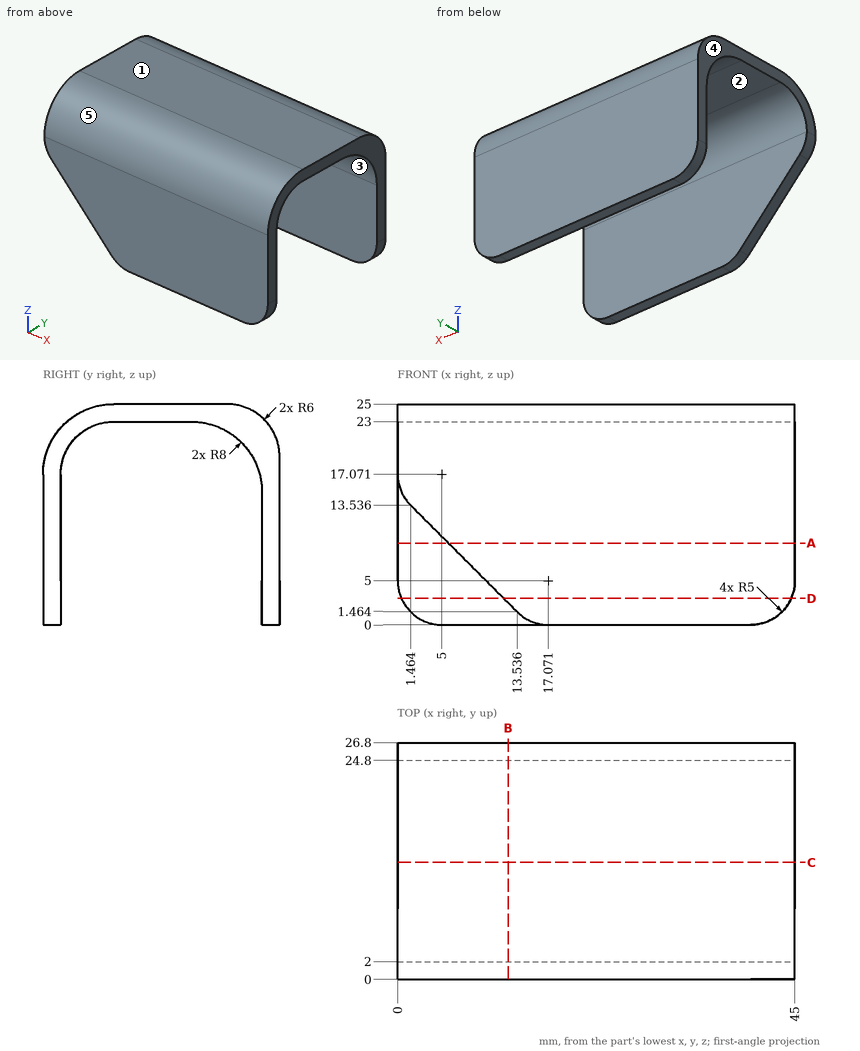
Here's the drawing with two shaded views (mm, measured from the low corner). I have some questions. A direction names the side the tool comes from. Give positions to 0.01 mm unless a question says otherwise; leave off trailing zeros. Loops run counter-clockwise (first coordinate to the right, second up) from the corner with the lowest first, then second, coordinate; pieces in that order, holes last. Notation, with made-up numbers: (47.5, 66.25) - (77.5, 66.25) arc R18 ccw to (77.5, 76.25) - close; hole circle Ø2 at (64, -12). An arc over 180 degrees is marked (long way). One line per item, written item: value.
(1) If we mould it in two halves opening along Y, with no side actions, what happens to the marked faces 3, 4 and 5? For each: released by +Y, released by -Y, zero draft, split by the parting line, or undercut.
Verdict:
face 3: undercut
face 4: zero draft
face 5: released by -Y
(2) If we section it at D-D, the plane z = 3: List the corners of the cut face in (x, y) for me.
Verdict:
outline: (0.42, 24.8) - (44.58, 24.8) - (44.58, 26.8) - (0.42, 26.8) - close; (12, 0) - (44.58, 0) - (44.58, 2) - (12, 2) - close
(3) If we section it at C-C, the plane y = 13.25: List the corners of the cut face in (x, z) for me.
Verdict:
outline: (0, 23) - (45, 23) - (45, 25) - (0, 25) - close
(4) On a 3-axis mill with a long thin cutter (end or side, diameter ignored), from which of +Z, -Z, +X, -X, +Y, -Y can I reach the whole of each face in a straight line? I mean the marked faces 1 and 2. Say none if no direction works.
Verdict:
face 1: +Z, +X, -X, +Y, -Y
face 2: -Z, +X, -X
(5) I need wall thicknesses on line 1 along Y through (x, z) = (28.5, 4.25); line 2 along Z through (x, y) = (8.5, 11.75); line 3 along Y through (x, z) = (25.5, 18.5) (1 decimal). Which ranges of each line are inside material? Lowest first, please.
Verdict:
line 1: 0 to 2, 24.8 to 26.8
line 2: 23 to 25
line 3: 0.1 to 2.2, 24 to 26.8
(6) If we section it at A-A, the plane z = 9.25: List the corners of the cut face in (x, y) for me.
Verdict:
outline: (0, 24.8) - (45, 24.8) - (45, 26.8) - (0, 26.8) - close; (5.75, 0) - (45, 0) - (45, 2) - (5.75, 2) - close
(7) I'm going to push flat-ended pins straight in: pin 1 (5 mm diameter, centred on x = 34, y = 21.5, fed in from -Z) (1 decimal); pin 2 (2.5 mm diameter, centred on x = 31.5, y = 12.5, fed in from -Z). Where does each tip first touch, or does it pass through?
Verdict:
pin 1: z = 18.5
pin 2: z = 23
(8) If we section it at B-B, the plane x = 12.5: List the corners of the cut face in (y, z) for me.
Verdict:
outline: (0, 2.5) - (2, 2.5) - (2, 17) arc R6 cw to (8, 23) - (16.8, 23) arc R8 cw to (24.8, 15) - (24.8, 0) - (26.8, 0) - (26.8, 19) arc R6 ccw to (20.8, 25) - (8, 25) arc R8 ccw to (0, 17) - close
